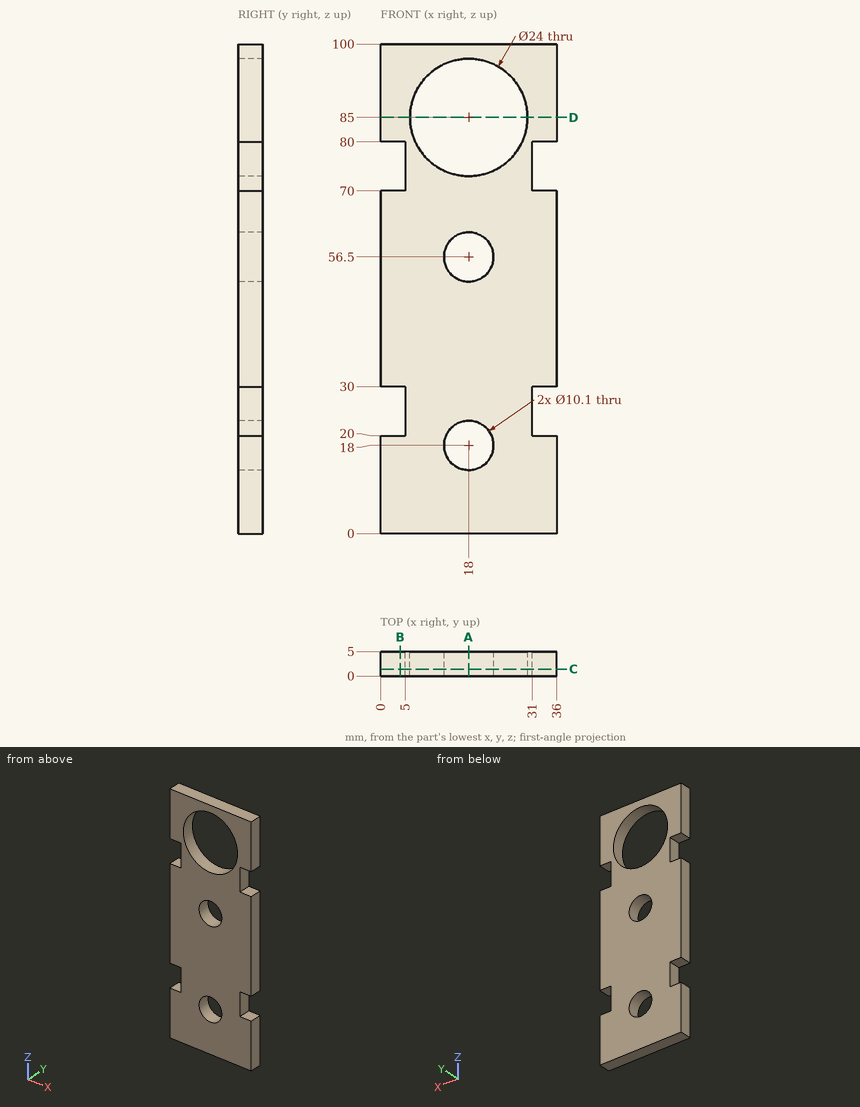
Study the drawing (mm; zero at the part's minimum x, y, z) and answer. Coordinates: 2 decimals unless noted, no trailing zeros. Write each loop counter-clockwise with the first axis right and the second up, starting at its lowest first coordinate (ties: lowest second). Pieces come first, ordered by that corner, then holes. Notation, with made-up numbers: (87.5, 79.5) -> (122.5, 79.5) arc R12 cw to (122.5, 100.5) -> close; hole circle Ø7 at (79, 45). An arc over 180 degrees is marked (long way). Write each question's results on one line, items separated by ' | '. Start each with the question number.
1) Straight lines are drawn through the part: probe 1 along Z at (x, y) = (32, 1.5); probe 2 along Z at (x, y) = (18, 1); probe 3 along X at (y, z) = (3.15, 56.5). For each, find the intervals that lie inside material, in ascending order.
2) A cutting plane is placed at B-B (x = 4). Determine the outline of the cut face in (y, z), then the cut area to 3 significant figures.
3) A cutting plane is placed at A-A (x = 18). Determine the outline of the cut face in (y, z), then the cut area to 3 significant figures.
4) A cutting plane is placed at D-D (z = 85). Determine the outline of the cut face in (x, y), then the cut area to 3 significant figures.
5) Flat-ended cylindrical pins translate along their axes: pin 1 Ø1.5 at (y, z) = (2.5, 25) entering from +X; pin 2 Ø1.5 at (y, z) = (1.5, 76) entering from -X. Find the tip coordinate at first contact, or state that the pin passes through.
6) A cutting plane is placed at C-C (y = 1.4). Determine the outline of the cut face in (x, z), then the cut area to 3 significant figures.
Values follow:
1) probe 1: 0 to 20, 30 to 70, 80 to 100 | probe 2: 0 to 12.95, 23.05 to 51.45, 61.55 to 73, 97 to 100 | probe 3: 0 to 12.95, 23.05 to 36
2) outline: (0, 0) -> (5, 0) -> (5, 20) -> (0, 20) -> close; (0, 30) -> (5, 30) -> (5, 70) -> (0, 70) -> close; (0, 80) -> (5, 80) -> (5, 100) -> (0, 100) -> close | area: 400 mm²
3) outline: (0, 0) -> (5, 0) -> (5, 12.95) -> (0, 12.95) -> close; (0, 23.05) -> (5, 23.05) -> (5, 51.45) -> (0, 51.45) -> close; (0, 61.55) -> (5, 61.55) -> (5, 73) -> (0, 73) -> close; (0, 97) -> (5, 97) -> (5, 100) -> (0, 100) -> close | area: 279 mm²
4) outline: (0, 0) -> (6, 0) -> (6, 5) -> (0, 5) -> close; (30, 0) -> (36, 0) -> (36, 5) -> (30, 5) -> close | area: 60.0 mm²
5) pin 1: x = 31 | pin 2: x = 5
6) outline: (0, 0) -> (36, 0) -> (36, 20) -> (31, 20) -> (31, 30) -> (36, 30) -> (36, 70) -> (31, 70) -> (31, 80) -> (36, 80) -> (36, 100) -> (0, 100) -> (0, 80) -> (5, 80) -> (5, 70) -> (0, 70) -> (0, 30) -> (5, 30) -> (5, 20) -> (0, 20) -> close; hole circle Ø24 at (18, 85); hole circle Ø10.1 at (18, 18); hole circle Ø10.1 at (18, 56.5) | area: 2,790 mm²
